Input: dimensioned drawing with shaded views. Units: mm. Origin: part minimum x, y, z. A direction names the side the tool comes from. Coordinates: 2 decimals unless noted, no trailing zeros. Order: outer loops, then holes, each group sorted by start corner. A loop starts at its lowest first (then second) coordinate and runs counter-clockwise, first axis right, second up.
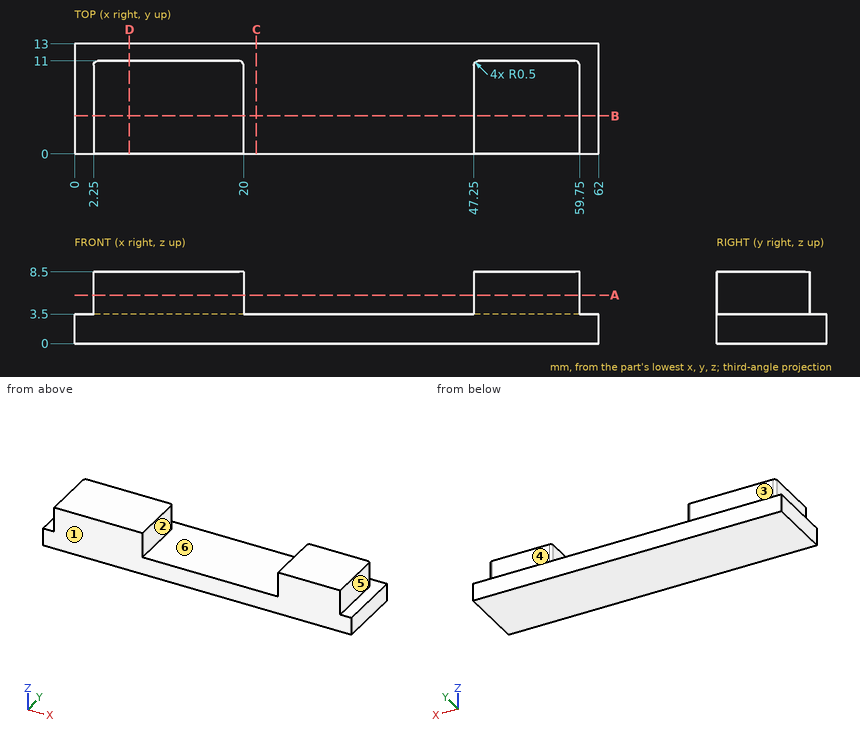
1. Pin query (flat end, axial travel): P1, Ø2.5, axis at y = 3, z = 6.5, coming from the +X side; P2, Ø2.5, axis at y = 5, z = 5, coming from the -X side; P3, Ø2.5, axis at x = 54, z = 6.5, coming from the +Y side. Return the tip coordinate at first contact, or that it passes through.
Findings:
P1: stops at x = 59.75
P2: stops at x = 2.25
P3: stops at y = 11
2. Section query C-C on x = 21.5. Return loops of the section in (y, z).
Findings:
outline: (0, 0) - (13, 0) - (13, 3.5) - (0, 3.5) - close
3. Access query for the marked faces 1, 2 and 3. Directions: +Z, -Z, +X, -X, +Y, -Y. A direction counts if a zero-diameter tool reaches every point of the face in a straight line with its end or side. Return the directions, or none.
Findings:
face 1: +Z, -Z, +X, -X, -Y
face 2: +Z, +Y, -Y
face 3: +Z, +X, -X, +Y
4. Section query B-B on y = 4.5. Return loops of the section in (x, z), plus the area to 3 significant figures.
Findings:
outline: (0, 0) - (62, 0) - (62, 3.5) - (59.75, 3.5) - (59.75, 8.5) - (47.25, 8.5) - (47.25, 3.5) - (20, 3.5) - (20, 8.5) - (2.25, 8.5) - (2.25, 3.5) - (0, 3.5) - close
area: 368 mm2
5. Section query A-A on z = 5.75. Return loops of the section in (x, y), plus the area to 3 significant figures.
Findings:
outline: (2.25, 0) - (20, 0) - (20, 10.5) arc R0.5 ccw to (19.5, 11) - (2.75, 11) arc R0.5 ccw to (2.25, 10.5) - close; (47.25, 0) - (59.75, 0) - (59.75, 10.5) arc R0.5 ccw to (59.25, 11) - (47.75, 11) arc R0.5 ccw to (47.25, 10.5) - close
area: 333 mm2
6. Section query D-D on x = 6.5. Return loops of the section in (y, z).
Findings:
outline: (0, 0) - (13, 0) - (13, 3.5) - (11, 3.5) - (11, 8.5) - (0, 8.5) - close
7. Ray query, line 1 (X direction, y = 10, z = 6); line 2 (Z direction, x = 43, y = 12). Return the intervals inside material, ascending.
Findings:
line 1: x = 2.25 to 20, 47.25 to 59.75
line 2: z = 0 to 3.5
8. Draft query along X for the marked faces 4, 5 and 6. Return one class per face: released by +X, released by -X, zero draft, split by the parting line, or undercut.
Findings:
face 4: zero draft
face 5: released by +X
face 6: undercut
